from build123d import *

# Parameters (mm, degrees)
BOSS_EXTRUDE1_DEPTH     = 17.5
SKETCH2_W               = 252
SKETCH2_H               = 14.5
CUT_EXTRUDE1_DEPTH      = 15.5
SKETCH3_R               = 13
CUT_EXTRUDE2_DEPTH      = 15.5
CUT_EXTRUDE3_REACH      = 264.265
CUT_EXTRUDE3_END_RADIUS = 13
SKETCH5_W               = 252
SKETCH5_H               = 1
BOSS_EXTRUDE2_DEPTH     = 2
SKETCH6_R               = 1
CUT_EXTRUDE4_DEPTH      = 2
CUT_EXTRUDE9_DEPTH      = 278.209870862


with BuildPart() as part:
    # Sketch1 → Boss-Extrude1 (new body)
    with BuildSketch(Plane(origin=(0, 0, 0), x_dir=(1, 0, 0), z_dir=(0, 1, 0))):
        with BuildLine():
            Line((0.323033708, 14.996521237), (267.19920412, 9.247854763))
            ThreePointArc((267.19920412, 9.247854763), (276.25, 0), (267.19920412, -9.247854763))
            Line((267.19920412, -9.247854763), (0.323033708, -14.996521237))
            ThreePointArc((0.323033708, -14.996521237), (-15, 0), (0.323033708, 14.996521237))
        make_face()
    extrude(amount=BOSS_EXTRUDE1_DEPTH)

    # Sketch2 → Cut-Extrude1 (cut)
    with BuildSketch(Plane(origin=(0, 17.5, 0), x_dir=(1, 0, 0), z_dir=(0, 1, 0))):
        with Locations((141, 0)):
            Rectangle(SKETCH2_W, SKETCH2_H)
    extrude(amount=-CUT_EXTRUDE1_DEPTH, mode=Mode.SUBTRACT)

    # Sketch3 → Cut-Extrude2 (cut)
    with BuildSketch(Plane(origin=(0, 17.5, 0), x_dir=(1, 0, 0), z_dir=(0, 1, 0))):
        with Locations(Location((0, 0, 0), (0, 0, 270))):
            Circle(SKETCH3_R)
    extrude(amount=-CUT_EXTRUDE2_DEPTH, mode=Mode.SUBTRACT)

    # Cut-Extrude3: up to this cylinder (the profile starts outside it)
    cut_extrude3_end = Plane(origin=(0, 8.125709, 0), z_dir=(0, 1, 0)) * Cylinder(CUT_EXTRUDE3_END_RADIUS, 555.53, mode=Mode.PRIVATE)
    # Sketch4 → Cut-Extrude3 (cut, up to the surface)
    with BuildSketch(Plane(origin=(15, 0, 0), x_dir=(0, 0, -1), z_dir=(1, 0, 0)), mode=Mode.PRIVATE) as cut_extrude3_sk1:
        with BuildLine():
            Line((-7.25, 2), (7.25, 2))
            Line((7.25, 2), (7.25, 8.5))
            ThreePointArc((7.25, 8.5), (5.199747468, 13.449747468), (0.25, 15.5))
            Line((0.25, 15.5), (-0.25, 15.5))
            ThreePointArc((-0.25, 15.5), (-5.199747468, 13.449747468), (-7.25, 8.5))
            Line((-7.25, 8.5), (-7.25, 2))
        make_face()
    cut_extrude3_tool1 = extrude(cut_extrude3_sk1.sketch, amount=-CUT_EXTRUDE3_REACH, mode=Mode.PRIVATE) - cut_extrude3_end
    add(cut_extrude3_tool1.solids().sort_by_distance((15, 8.125709, 0))[0], mode=Mode.SUBTRACT)

    # Sketch5 → Boss-Extrude2 (add)
    with BuildSketch(Plane(origin=(0, 2, 0), x_dir=(1, 0, 0), z_dir=(0, 1, 0))):
        with Locations((141, 6.75)):
            Rectangle(SKETCH5_W, SKETCH5_H)
        with Locations((141, -6.75)):
            Rectangle(SKETCH5_W, SKETCH5_H)
    extrude(amount=BOSS_EXTRUDE2_DEPTH)

    # Sketch6 → Cut-Extrude4 (cut)
    with BuildSketch(Plane(origin=(0, 2, 0), x_dir=(1, 0, 0), z_dir=(0, 1, 0))):
        with Locations(Location((-5.25, 9.09326674, 0), (0, 0, 270))):
            Circle(SKETCH6_R)
        with Locations(Location((-10.5, 0, 0), (0, 0, 270))):
            Circle(SKETCH6_R)
        with Locations(Location((5.25, 9.09326674, 0), (0, 0, 270))):
            Circle(SKETCH6_R)
        with Locations(Location((10.5, 0, 0), (0, 0, 270))):
            Circle(SKETCH6_R)
        with Locations(Location((5.25, -9.09326674, 0), (0, 0, 270))):
            Circle(SKETCH6_R)
        with Locations(Location((-5.25, -9.09326674, 0), (0, 0, 270))):
            Circle(SKETCH6_R)
        Polygon((0, -10), (8.660254038, -5), (8.660254038, 5), (0, 10), (-8.660254038, 5), (-8.660254038, -5), align=None)
    extrude(amount=-CUT_EXTRUDE4_DEPTH, mode=Mode.SUBTRACT)

    # Sketch14 → Cut-Extrude9 (cut, through all)
    with BuildSketch(Plane(origin=(0, 0, 0), x_dir=(1, 0, 0), z_dir=(0, 1, 0))):
        Polygon((88.5, 9.35), (78.6, 9.35), (78.6, 35), (78.4, 35), (78.4, 9.15), (88.3, 9.15), (88.3, -9.15), (78.4, -9.15), (78.4, -35), (78.6, -35), (78.6, -9.35), (88.5, -9.35), align=None)
        Polygon((172.7, 9.15), (182.6, 9.15), (182.6, 35), (182.4, 35), (182.4, 9.35), (172.5, 9.35), (172.5, 9.25), (172.5, -9.35), (182.4, -9.35), (182.4, -35), (182.6, -35), (182.6, -9.15), (172.7, -9.15), align=None)
    extrude(amount=CUT_EXTRUDE9_DEPTH, mode=Mode.SUBTRACT)


with BuildPart() as cut_extrude9_kept_piece:
    # of the separate pieces the step leaves, the one the design keeps (cut_extrude9_pieces_kept)
    add(part.part.solids().sort_by_distance((267.19920412, 0, 9.247854763))[0])


solid = cut_extrude9_kept_piece.part
The listing builds one solid part. Answer for the finished solid, in the listing's coordinates (mm). A direction names the side the tool comes from. Give positions to 0.01 mm unless a question says otherwise; leave off trailing zeros. Write each loop counter-clockwise with the first axis right and the second up, starting at its lowest first coordinate (ties: lowest second). Pieces come first, ordered by that corner, then holes. Notation, with made-up numbers: (46, 61) - (80, 61) arc R22 ccw to (80, 70) - close; hole circle Ø4 at (10, 38). An arc over 180 degrees is marked (long way). Use a Markdown table: item, result.
1. For a pull along Z with two mould halves and no side action, classify faces 1 (the flat face through (178, 9, -9.15)), 2 (the flat face through (219, 3, -6.25)), 3 (the flat face through (225, 0, 0)) as released by +Z, released by -Z, zero draft, split by the parting line, or undercut.
Values follow:
| item | result |
|---|---|
| face 1 | released by -Z |
| face 2 | undercut |
| face 3 | zero draft |
2. Section C-C on z = 0 is taken. Write down the section's boundary in (x, y), plus the area to 3 significant figures.
Values follow:
| item | result |
|---|---|
| outline | (172.7, 0) - (276.25, 0) - (276.25, 17.5) - (267, 17.5) - (267, 2) - (172.7, 2) - close |
| area | 350 mm² |
3. Find the intervals of material crossed by probe 1 along Z at (x, y) = (182.5, 3.5); probe 2 along Z at (x, y) = (264, 5.75); probe 3 along Y at (x, z) = (226.5, 1), in increasing order. Write a range as from..to.
Values follow:
| item | result |
|---|---|
| probe 1 | z = -9.15..-6.25, 6.25..9.15 |
| probe 2 | z = -9.32..-7.25, 7.25..9.32 |
| probe 3 | y = 0..2 |
4. Section A-A on y = 6 is taken. Write down the section's boundary in (x, z), plus the area to 3 significant figures.
Values follow:
| item | result |
|---|---|
| outline | (172.7, -9.15) - (182.6, -9.15) - (182.6, -11.07) - (267.2, -9.25) arc R9.25 ccw to (267.2, 9.25) - (182.6, 11.07) - (182.6, 9.15) - (172.7, 9.15) - (172.7, 7.25) - (267, 7.25) - (267, -7.25) - (172.7, -7.25) - close |
| area | 663 mm² |
5. A tool of negligible diameter and unlimited length cuts with its end or side. For faces 4 (the flat face through (219, 3, 6.25)), 5 (the flat face through (178, 9, 9.15)), 6 (the flat face through (182.6, 9, -10)), from which of +Z, -Z, +X, -X, +Y, -Y can it reach the whole face along a straight path? Write none if from no direction.
Values follow:
| item | result |
|---|---|
| face 4 | -X, +Y |
| face 5 | +Z, -X, +Y, -Y |
| face 6 | -Z, -X, +Y, -Y |
6. Section B-B on x = 230 is taken. Write down the section's boundary in (y, z), plus the area to 3 significant figures.
Values follow:
| item | result |
|---|---|
| outline | (0, -10.05) - (17.5, -10.05) - (17.5, -7.25) - (4, -7.25) - (4, -6.25) - (2, -6.25) - (2, 6.25) - (4, 6.25) - (4, 7.25) - (17.5, 7.25) - (17.5, 10.05) - (0, 10.05) - close |
| area | 131 mm² |
7. Each of these flat-tipped pins is pushed along its axis until it touches: P1, Ø0.5, axis at x = 241, z = 6.5, coming from the +Y side; P2, Ø4, axis at y = 7, z = -2, coming from the -X side; P3, Ø0.6, axis at y = 5.5, z = 10, coming from the -X side. Where does it stop, or does it pass through?
Values follow:
| item | result |
|---|---|
| P1 | stops at y = 4 |
| P2 | stops at x = 267 |
| P3 | stops at x = 182.6 |
